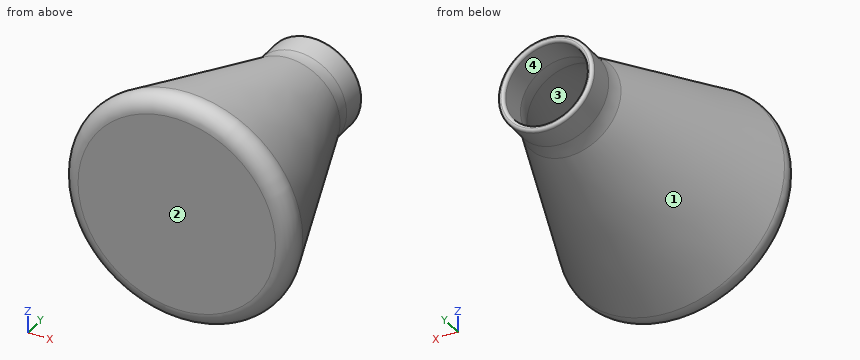
from build123d import *

# Parameters (mm, degrees)
SHELL1_T                  = -8
SHELL1_THICKNESS_2_FACE_R = 141.387225684
SHELL1_THICKNESS_2_DEPTH  = 4
FILLET1_R                 = 4
FILLET2_R                 = 60
FILLET3_R                 = 20


with BuildPart() as part:
    # Sketch1 → Revolve2 (revolve)
    with BuildSketch(Plane.XY, mode=Mode.PRIVATE) as revolve2_sk:
        Polygon((0, 0), (0, 300), (60, 300), (60, 255), (152.812409738, 0), align=None)
    revolve(revolve2_sk.sketch.rotate(Axis((0, 0, 0), (0, 1, 0)), 90), axis=Axis((0, 0, 0), (0, 1, 0)))

    # Shell1
    shell1_openings = [part.faces().sort_by_distance(p)[0] for p in [
        (0, 300, 0),
    ]]
    offset(amount=SHELL1_T, openings=shell1_openings, kind=Kind.INTERSECTION)

    # Shell1 thickness 2 face (on inner face of the shell) → Shell1 thickness 2 (add)
    with BuildSketch(Plane(origin=(0, 8, 0), x_dir=(0, 0, -1), z_dir=(0, -1, 0))):
        Circle(SHELL1_THICKNESS_2_FACE_R)
    extrude(amount=-SHELL1_THICKNESS_2_DEPTH)

    # Fillet1
    fillet1_edges = [part.edges().sort_by_distance(p)[0] for p in [
        (0, 300, 52),
        (0, 300, 60),
    ]]
    fillet(fillet1_edges, radius=FILLET1_R - 0.0001)  # a hair under: the kernel refuses the full size

    # Fillet2
    fillet2_edges = [part.edges().sort_by_distance(p)[0] for p in [
        (0, 253.589384154, 52),
        (0, 255, 60),
    ]]
    fillet(fillet2_edges, radius=FILLET2_R)

    # Fillet3
    fillet3_edges = [part.edges().sort_by_distance(p)[0] for p in [
        (0, 12, 139.931344747),
        (0, 0, 152.812409738),
    ]]
    fillet(fillet3_edges, radius=FILLET3_R)


solid = part.part
Part model, mm, in its own coordinate system. Face numbers are marked on the shaded views. Coordinates: 2 decimals unless noted, no trailing zeros. Order: outer loops, then holes, each group sorted by start corner. A loop starts at its lowest first (then second) coordinate and runs counter-clockwise, first axis right, second up.
(1) Slice it at B-B, the plane y = 130.5. Write the cut outline in (x, z).
Check sheet entries:
outline: circle Ø210.63 at (0, 0); hole circle Ø193.6 at (0, 0)
(2) Pin check, flat tips, straight feed: pin 1 Ø12 at (y, z) = (102, 90) entering from +X; pin 2 Ø1.5 at (y, z) = (68.5, -45.5) entering from -X. Stop position of each tip, or through.
Check sheet entries:
pin 1: stops at x = 80.3
pin 2: stops at x = -119.92
(3) Slice it at A-A, the plane y = 209. Write the cut outline in (x, z), and give its area (3 significant figures).
Check sheet entries:
outline: circle Ø153.49 at (0, 0); hole circle Ø136.46 at (0, 0)
area: 3,880 mm2
(4) Pull direction X, two halves, no side cores. Call the marked faces 1, 2, 3 and 4: pulls with the +X half, pulls with the -X half, needs draft (parallel to the pull), parting line crosses it, or undercut.
Check sheet entries:
face 1: parting line crosses it
face 2: needs draft
face 3: undercut
face 4: undercut
(5) Probe L1, parallel to X at y = 272, z = 0; L2, parallel to Y at x = -44.5, z = -79.5; L3, parallel to Z at x = -11, y = 120. List the from-to ranges inside material, lowest first.
Check sheet entries:
L1: x = -60 to -52, 52 to 60
L2: y = 0 to 12, 146.14 to 169.53
L3: z = -108.58 to -100.02, 100.02 to 108.58
